Here's the drawing with two shaded views (mm, measured from the low corner). I have some questions. A direction names the side the tool comes from. Give positions to 0.01 mm unless a question says otherwise; leave off trailing zeros. Loops run counter-clockwise (first coordinate to the right, second up) from the corner with the lowest first, then second, coordinate; pieces in that order, holes last. Notation, with made-up numbers: M -9.5,50 L 1.5,50 A23 cw 1.5,72 Z; hole C 20,20 d9. An arc over 180 degrees is marked long. Answer in a Markdown table with one row per item. Add a question column.
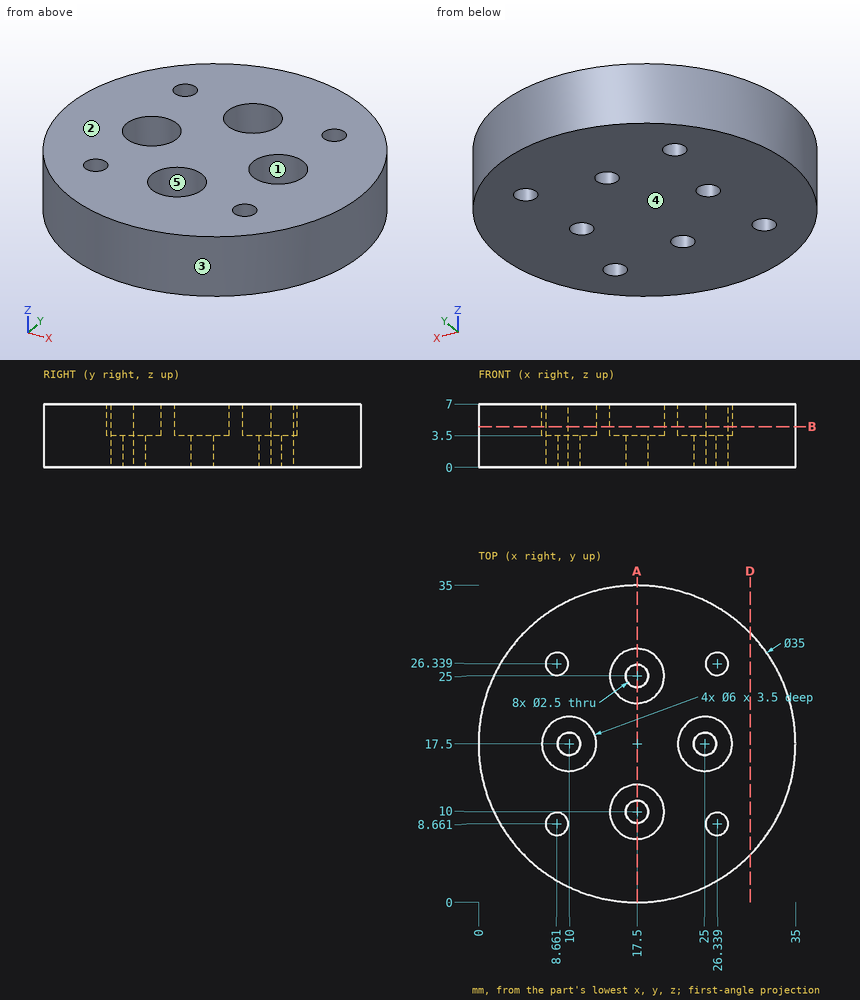
Item 1: Suppose I cut it at B-B (z = 4.5). Give the number of separate pieces and of enclosed holes in the cut face, then the cut area to 3 significant figures.
Item 2: Suppose I cut it at A-A (x = 17.5). List the corners of the cut face in (y, z) for me.
Item 3: I need wall thicknesses on L1, parallel to Y at x = 17.5, z = 5.2; L2, parallel to Y at x = 17.5, z = 2.7; L3, parallel to X at y = 31.5, z = 1.25. Which ranges of each line are inside material? Lowest first, please.
Item 4: Suppose I cut it at D-D (x = 30). List the corners of the cut face in (y, z) for me.
Item 5: For P1, Ø1.8, axis at x = 8.5, y = 17, coming from the +Z side; P2, Ø2, axis at x = 6, z = 4.5, coming from the -Y side, each with a flat end and sliding along its axis, tell me the tip position at first contact or that it passes through.
Item 6: For the marked faces 1 and 2, which set-ups out of +Z, -Z, +X, -X, +Y, -Y let a thin tool reach every point of the face, with its end or its side?
Item 7: If we mould it in two halves opening along X, with no side actions, what happens to the marked faces 3, 4 and 5? For each: +X half, -X half, draft (parallel to the pull), parting line (faces both ways), or undercut.
Values found:
| question | item | result |
|---|---|---|
| 1 | separate pieces | 1 |
| 1 | enclosed holes | 8 |
| 1 | area | 829 mm² |
| 2 | outline | M 0,0 L 8.75,0 L 8.75,3.5 L 7,3.5 L 7,7 L 0,7 Z; M 11.25,0 L 23.75,0 L 23.75,3.5 L 22,3.5 L 22,7 L 13,7 L 13,3.5 L 11.25,3.5 Z; M 26.25,0 L 35,0 L 35,7 L 28,7 L 28,3.5 L 26.25,3.5 Z |
| 3 | L1 | 0 to 7, 13 to 22, 28 to 35 |
| 3 | L2 | 0 to 8.75, 11.25 to 23.75, 26.25 to 35 |
| 3 | L3 | 7 to 28 |
| 4 | outline | M 5.25,0 L 29.75,0 L 29.75,7 L 5.25,7 Z |
| 5 | P1 | z = 3.5 |
| 5 | P2 | y = 3.5 |
| 6 | face 1 | +Z |
| 6 | face 2 | +Z, +X, -X, +Y, -Y |
| 7 | face 3 | parting line |
| 7 | face 4 | draft |
| 7 | face 5 | undercut |
